For this review, take the finished solid that the model builds, in its own axes (mm). Coordinates: 2 decimals unless noted, no trailing zeros. Write each loop counter-clockwise with the first axis right and the second up, starting at its lowest first coordinate (ties: lowest second). Pieces come first, ordered by that corner, then holes. Notation, with made-up numbers: (75, 40.25) -> (128, 40.25) arc R23 cw to (128, 78.25) -> close; hole circle Ø9 at (-32.75, -18.5). An arc over 180 degrees is marked (long way). One line per item, written item: value. Start each with the question number.
1) Add section A-A (y = 2.6). State the section outline as (x, z) points, and give its area (3 significant figures).
2) Mouldability with a two-part tool opening along Z and no side actions: class faces 1 (the flat face through (-20, 3, 16.585)), 2 (the flat face through (-54.915, 3, 18)), 3 (the cylindrical face through (-54.1, 2.6, 18.5)) as released by +Z, released by -Z, zero draft, split by the parting line, or undercut.
3) For probe 1 along X at (y, z) = (0.95, 18.8); probe 2 along Y at (x, z) = (-18, 17.9); probe 3 along X at (y, z) = (0.7, 18.4), list the stretches that pass through material, from the lowest coordinate up. Write a range as from..to.
4) Add section C-C (x = -19). State the section outline as (y, z) points, and give its area (3 significant figures).
5) For pin 1 Ø1.5 at (x, z) = (-23.5, 18.5) entering from -Y, flat-tipped, find the tip position at first contact; note if it passes through.
6) Add section B-B (z = 18.25). State the section outline as (x, y) points, and give its area (3 significant figures).
from build123d import *

# Parameters (mm, degrees)
SKETCH1_W           = 71
SKETCH1_H           = 3
BOSS_EXTRUDE1_DEPTH = 5.2
SKETCH2_R           = 0.8
CUT_EXTRUDE1_DEPTH  = 5.2
SKETCH3_R           = 1.6
CUT_EXTRUDE2_DEPTH  = 5.2


with BuildPart() as part:
    # Sketch1 → Boss-Extrude1 (new body)
    with BuildSketch(Plane(origin=(0, 0, 0), x_dir=(1, 0, 0), z_dir=(0, 1, 0))):
        with Locations((-19.414749289, -18.085343374)):
            Rectangle(SKETCH1_W, SKETCH1_H)
    extrude(amount=BOSS_EXTRUDE1_DEPTH)

    # Sketch2 → Cut-Extrude1 (cut)
    with BuildSketch(Plane(origin=(0, 5.2, 0), x_dir=(1, 0, 0), z_dir=(0, 1, 0))):
        with Locations(Location((-53.414749289, -18.085343374, 0), (0, 0, 270))):
            Circle(SKETCH2_R)
        with Locations(Location((14.585250711, -18.085343374, 0), (0, 0, 270))):
            Circle(SKETCH2_R)
    extrude(amount=-CUT_EXTRUDE1_DEPTH, mode=Mode.SUBTRACT)

    # Sketch3 → Cut-Extrude2 (cut)
    with BuildSketch(Plane(origin=(0, 0, 16.585343374), x_dir=(-1, 0, 0), z_dir=(0, 0, -1))):
        with Locations((18.164749289, 2.6)):
            Circle(SKETCH3_R)
    extrude(amount=-CUT_EXTRUDE2_DEPTH, mode=Mode.SUBTRACT)


solid = part.part
Numbers:
1. outline: (-54.91, 16.59) -> (-19.76, 16.59) -> (-19.76, 19.59) -> (-54.91, 19.59) -> close; (-16.56, 16.59) -> (16.09, 16.59) -> (16.09, 19.59) -> (-16.56, 19.59) -> close; hole circle Ø1.6 at (-53.41, 18.09); hole circle Ø1.6 at (14.59, 18.09)
1. area: 199 mm²
2. face 1: released by -Z
2. face 2: zero draft
2. face 3: undercut
3. probe 1: -54.91..-53.77, -53.06..14.23, 14.94..16.09
3. probe 2: 0..1.01, 4.19..5.2
3. probe 3: -54.91..-54.15, -52.68..13.85, 15.32..16.09
4. outline: (0, 16.59) -> (1.24, 16.59) -> (1.24, 19.59) -> (0, 19.59) -> close; (3.96, 16.59) -> (5.2, 16.59) -> (5.2, 19.59) -> (3.96, 19.59) -> close
4. area: 7.41 mm²
5. pin 1: y = 0
6. outline: (-54.91, 0) -> (-54.2, 0) -> (-54.2, 5.2) -> (-54.91, 5.2) -> close; (-52.63, 0) -> (13.8, 0) -> (13.8, 5.2) -> (-52.63, 5.2) -> close; (15.37, 0) -> (16.09, 0) -> (16.09, 5.2) -> (15.37, 5.2) -> close; hole circle Ø3.2 at (-18.16, 2.6)
6. area: 345 mm²
